Read the model definition and answer for the solid it produces. Units are mm, in the model's axes. Face numbers are marked on the shaded views. A direction names the side the tool comes from. Coordinates: 2 decimals unless noted, no trailing zeros. Write each loop counter-clockwise with the first axis right and the second up, starting at its lowest first coordinate (ties: lowest second). Pieces come first, ordered by that corner, then holes.
(1) Section B-B on z = 2 is taken. Write down the section's boundary in (x, y).
(2) Find the intervals of material crossed by probe 1 along Y at (x, z) = (0, 3.5); probe 2 along Y at (x, z) = (0, 39.75); probe 3 along Z at (x, y) = (31, 21.5), in increasing order.
(3) The mould has two halves that part along Y. Classify the marked faces 3, 4 and 5: +Y half, -Y half, draft (parallel to the pull), parting line (faces both ways), or undercut.
(4) Which of the six approach directions +Z, -Z, +X, -X, +Y, -Y give full straight-line access (tool end or side, diameter ignored) to the marked faces 1 and 2?
(5) Given pin 1 (2 mm diameter, centred on x = 19.5, y = -0.5, fed in from +Z); pin 2 (4 mm diameter, centred on y = -14, z = 10.5, fed in from +X); pin 3 (5 mm diameter, centred on x = -19.5, y = 23.5, fed in from -Z), each flat-ended and moving along its own axis, determine where each tip first touches the part or whether it passes through.
(6) Section A-A on z = 35.5 is taken. Write down the section's boundary in (x, y), then the cut area to 3 significant figures.
(7) Section C-C on x = -24.5 is taken. Write down the section's boundary in (y, z), then the cut area to 3 significant figures.
(8) Section D-D on y = -4 is taken. Write down the section's boundary in (x, z), then the cut area to 3 significant figures.
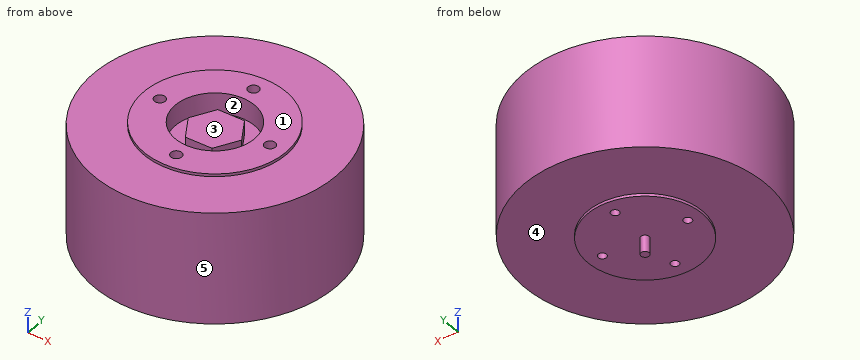
from build123d import *

# Parameters (mm, degrees)
SKETCH_1_R               = 44.25
EXTRUDE_1_DEPTH          = 41
SKETCH_2_R               = 26
EXTRUDE_2_DEPTH          = 1
SKETCH_3_R               = 2
CUT_EXTRUDE_1_DEPTH      = 10
SKETCH_5_R               = 21
EXTRUDE_4_DEPTH          = 1
SKETCH_6_R               = 1.5
CUT_EXTRUDE_2_DEPTH      = 10
PATTERN_CIRCULAR_1_COUNT = 4
SKETCH_7_R               = 1.5
EXTRUDE_5_DEPTH          = 6
SKETCH_8_R               = 14.5
CUT_EXTRUDE_3_DEPTH      = 7.6
EXTRUDE_6_DEPTH          = 5


with BuildPart() as part:
    # 草图1 → 凸台-拉伸1 (new body)
    with BuildSketch(Plane.XY):
        Circle(SKETCH_1_R)
    extrude(amount=EXTRUDE_1_DEPTH)

    # 草图2 → 凸台-拉伸2 (add)
    with BuildSketch(Plane.XY.offset(41)):
        Circle(SKETCH_2_R)
    extrude(amount=EXTRUDE_2_DEPTH)

    # 草图3 → 切除-拉伸1 (cut)
    with BuildSketch(Plane.XY.offset(42)):
        with Locations((0, 20)):
            Circle(SKETCH_3_R)
        with Locations((20, 0)):
            Circle(SKETCH_3_R)
        with Locations((0, -20)):
            Circle(SKETCH_3_R)
        with Locations((-20, 0)):
            Circle(SKETCH_3_R)
    extrude(amount=-CUT_EXTRUDE_1_DEPTH, mode=Mode.SUBTRACT)

    # 草图5 → 凸台-拉伸4 (add)
    with BuildSketch(Plane(origin=(0, 0, 0), x_dir=(-1, 0, 0), z_dir=(0, 0, -1))):
        Circle(SKETCH_5_R)
    extrude(amount=EXTRUDE_4_DEPTH)

    # 草图6 → 切除-拉伸2 (cut)
    with BuildSketch(Plane(origin=(0, 0, -1), x_dir=(-1, 0, 0), z_dir=(0, 0, -1))):
        with Locations((0, 15.5)):
            Circle(SKETCH_6_R)
    cut_extrude_2 = extrude(amount=-CUT_EXTRUDE_2_DEPTH, mode=Mode.SUBTRACT)

    # 阵列(圆周)1: 切除-拉伸2 ×4 about axis
    pattern_circular_1_axis = Axis((0, 0, 0), (0, 0, 1))
    for i in range(1, PATTERN_CIRCULAR_1_COUNT):
        add(cut_extrude_2.rotate(pattern_circular_1_axis, i * 360 / PATTERN_CIRCULAR_1_COUNT), mode=Mode.SUBTRACT)

    # 草图7 → 凸台-拉伸5 (add)
    with BuildSketch(Plane(origin=(0, 0, -1), x_dir=(-1, 0, 0), z_dir=(0, 0, -1))):
        Circle(SKETCH_7_R)
    extrude(amount=EXTRUDE_5_DEPTH)

    # 草图8 → 切除-拉伸3 (cut)
    with BuildSketch(Plane.XY.offset(42)):
        Circle(SKETCH_8_R)
    extrude(amount=-CUT_EXTRUDE_3_DEPTH, mode=Mode.SUBTRACT)

    # 草图9 → 凸台-拉伸6 (add)
    with BuildSketch(Plane.XY.offset(34.4)):
        Polygon((9.699484522, 0), (4.849742261, 8.4), (-4.849742261, 8.4), (-9.699484522, 0), (-4.849742261, -8.4), (4.849742261, -8.4), align=None)
    extrude(amount=EXTRUDE_6_DEPTH)


solid = part.part
Response:
1. outline: circle Ø88.5 at (0, 0); hole circle Ø3 at (-15.5, 0); hole circle Ø3 at (0, -15.5); hole circle Ø3 at (0, 15.5); hole circle Ø3 at (15.5, 0)
2. probe 1: y = -44.25 to -17, -14 to 14, 17 to 44.25
2. probe 2: y = -44.25 to -22, -18 to -14.5, 14.5 to 18, 22 to 44.25
2. probe 3: z = 0 to 41
3. face 3: undercut
3. face 4: draft
3. face 5: parting line
4. face 1: +Z, +X, -X, +Y, -Y
4. face 2: +Z
5. pin 1: stops at z = 32
5. pin 2: stops at x = 42.59
5. pin 3: stops at z = 0
6. outline: circle Ø88.5 at (0, 0); (-9.7, 0) - (-4.85, -8.4) - (4.85, -8.4) - (9.7, 0) - (4.85, 8.4) - (-4.85, 8.4) - close; hole circle Ø4 at (-20, 0); hole circle Ø29 at (0, 0); hole circle Ø4 at (0, -20); hole circle Ø4 at (0, 20); hole circle Ø4 at (20, 0)
6. area: 5,690 mm2
7. outline: (-36.85, 0) - (36.85, 0) - (36.85, 41) - (8.7, 41) - (8.7, 42) - (-8.7, 42) - (-8.7, 41) - (-36.85, 41) - close
7. area: 3,040 mm2
8. outline: (-44.07, 0) - (-20.62, 0) - (-20.62, -1) - (20.62, -1) - (20.62, 0) - (44.07, 0) - (44.07, 41) - (25.69, 41) - (25.69, 42) - (13.94, 42) - (13.94, 34.4) - (7.39, 34.4) - (7.39, 39.4) - (-7.39, 39.4) - (-7.39, 34.4) - (-13.94, 34.4) - (-13.94, 42) - (-25.69, 42) - (-25.69, 41) - (-44.07, 41) - close
8. area: 3,570 mm2
